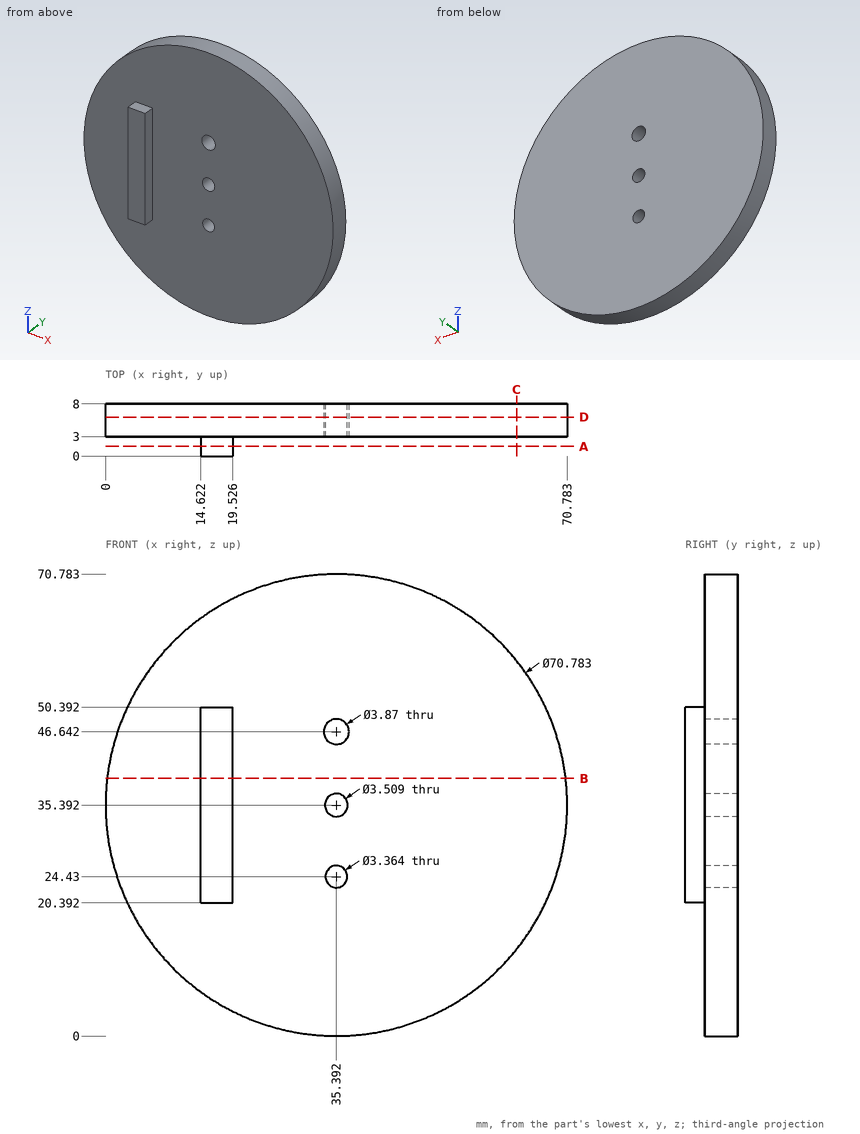
Check sheet for the drawn part. Datum: minimum x, y, z corner. Units: mm. Give positions to 0.01 mm unless a question says otherwise; leave off trailing zeros. Write each loop counter-clockwise with the first axis right and the second up, starting at its lowest first coordinate (ties: lowest second). Pieces come first, ordered by that corner, then holes. Notation, with made-up numbers: (50.25, 43.25) -> (108.25, 43.25) arc R34 ccw to (108.25, 80.25) -> close; hole circle Ø6 at (88.25, 13). An arc over 180 degrees is marked (long way). Use one line per item in the form item = value. Start each with the question number.
1. Section check B-B (z = 39.5). Record the cut outline in (x, y).
2. Thickness scan on line 1 along Y through (x, z) = (30, 55); line 2 along Z through (x, y) = (15, 2.5); line 3 along X through (y, z) = (4.5, 52) (1 decimal). Record the ranges inside material, lowest first. Write a range as from..to.
3. Section check C-C (x = 63). Record the cut outline in (y, z) (1 decimal).
4. Section check D-D (y = 6). Record the cut outline in (x, z) (1 decimal), and give its area (3 significant figures).
5. Go/stop test with flat-tipped pins: P1, Ø4, axis at y = 3, z = 63, coming from the +X side; P2, Ø2, axis at x = 47.5, z = 17.5, coming from the -Y side; P3, Ø2.5, axis at y = 1, z = 34.5, coming from the +X side. Record where each tip stops, or that it passes through.
6. Section check A-A (y = 1.5). Record the cut outline in (x, z).
Conclusion:
q1.outline = (0.24, 3) -> (14.62, 3) -> (14.62, 0) -> (19.53, 0) -> (19.53, 3) -> (70.54, 3) -> (70.54, 8) -> (0.24, 8) -> close
q2.line_1 = 3..8
q2.line_2 = 20.39..50.39
q2.line_3 = 4.1..66.6
q3.outline = (3, 13.2) -> (8, 13.2) -> (8, 57.5) -> (3, 57.5) -> close
q4.outline = circle Ø70.8 at (35.4, 35.4); hole circle Ø3.9 at (35.4, 46.6); hole circle Ø3.5 at (35.4, 35.4); hole circle Ø3.4 at (35.4, 24.4)
q4.area = 3,900 mm²
q5.P1 = 59.82
q5.P2 = 3
q5.P3 = 19.53
q6.outline = (14.62, 20.39) -> (19.53, 20.39) -> (19.53, 50.39) -> (14.62, 50.39) -> close
